Geometry check sheet. Reference: the model listing, model coordinates, mm. A direction names the side the tool comes from. Round coordinates to 2 decimals unless told otherwise and drop trailing zeros. Order: outer loops, then holes, each group sorted by start corner. A loop starts at its lowest first (then second) coordinate and runs counter-clockwise, first axis right, second up. Notation, with made-up numbers: (64.5, 13) -> (97.5, 13) arc R24 cw to (97.5, 44) -> close; hole circle Ø7 at (-4, 45.5). An arc over 180 degrees is marked (long way). Answer as a JSON object with one key per item and string values. Group by question number.
Autodesk Inventor part; units mm, degrees
ref_plane "YZ Plane" through (0, 0, 0) normal (1, 0, 0) x (0, 1, 0)
ref_plane "XZ Plane" through (0, 0, 0) normal (0, 1, 0) x (-1, 0, 0)
ref_plane "XY Plane" through (0, 0, 0) normal (0, 0, 1) x (1, 0, 0)
sketch "Sketch1" plane through (0, 0, 0) normal (0, 0, 1) x (1, 0, 0)
  line L0 (-35.56, 0) -> (35.56, 0) construction
  line L1 (0, -35.56) -> (0, 35.56) construction
  line L2 (-25.4, 25.4) -> (25.4, 25.4)
  line L3 (25.4, 25.4) -> (25.4, -25.4)
  line L4 (25.4, -25.4) -> (-25.4, -25.4)
  line L5 (-25.4, -25.4) -> (-25.4, 25.4)
  line L6 (-22.225, 22.225) -> (22.225, 22.225)
  line L7 (22.225, 22.225) -> (22.225, -22.225)
  line L8 (22.225, -22.225) -> (-22.225, -22.225)
  line L9 (-22.225, -22.225) -> (-22.225, 22.225)
  point P0 (0, 0)
  point P1 (-25.4, 0)
  point P2 (0, 25.4)
  point P3 (-22.225, 0)
  point P4 (0, 22.225)
  dimension "d0" = 50.8
  dimension "d1" = 3.175
  dimension "d11" = 50.8
  dimension "d12" = 3.175
extrude "Extrusion1" add sketch "Sketch1" along normal mid plane 101.6
sketch "Sketch6" plane through (-25.4, -25.4, 50.8) normal (-1, 0, 0) x (0, 0, 1)
  line L0 (-121.92, 25.4) -> (20.32, 25.4) construction
  line L1 (-50.8, -10.16) -> (-50.8, 60.96) construction
  line L2 (-71.8058, 50.8) -> (-29.7942, 50.8)
  line L3 (-29.7942, 50.8) -> (-29.7942, 0)
  line L4 (-29.7942, 0) -> (-71.8058, 0)
  line L5 (-71.8058, 0) -> (-71.8058, 50.8)
  line L6 (-101.6, 50.8) -> (0, 50.8) construction
  point P0 (-50.8, 25.4)
  point P1 (-71.8058, 25.4)
  point P2 (-50.8, 50.8)
  dimension "d23" = 42.0116
extrude "Extrusion7" cut sketch "Sketch6" against normal blind 3.175
sketch "Sketch7" plane through (-25.4, 25.4, 50.8) normal (0, 1, 0) x (1, 0, 0)
  circle A0 centre (37.35, 38.1) radius 2.0193 construction
  circle A1 centre (37.35, 63.5) radius 2.0193 construction
  circle A2 centre (37.35, 63.5) radius 2.413
  circle A3 centre (37.35, 38.1) radius 2.413
  point P0 (25.4, 50.8)
  dimension "d39" = 4.826
sketch "Sketch8" plane through (25.4, -25.4, 50.8) normal (1, 0, 0) x (0, 0, -1)
  line L0 (43.6, 4.4) -> (58, 4.4) construction
  line L1 (58, 4.4) -> (59.225, 3.175) construction
  line L2 (59.225, 3.175) -> (64.8, 3.175) construction
  line L3 (64.8, 9.4) -> (64.8, 3.175) construction
  arc A0 (66.8, 11.4) -> (64.8, 9.4) centre (66.8, 9.4) ccw construction
  line L4 (71.8, 11.4) -> (66.8, 11.4) construction
  line L5 (71.8, 11.4) -> (71.8, 45.4) construction
  arc A1 (71.8, 45.4) -> (70.8, 46.4) centre (50.8, 25.4) ccw construction
  line L6 (70.8, 46.4) -> (69, 46.4) construction
  line L7 (69, 46.4) -> (67.775, 47.625) construction
  line L8 (67.775, 47.625) -> (59.225, 47.625) construction
  line L9 (59.225, 47.625) -> (58, 46.4) construction
  line L10 (58, 46.4) -> (43.6, 46.4) construction
  line L11 (43.6, 46.4) -> (42.375, 47.625) construction
  line L12 (42.375, 47.625) -> (36.8, 47.625) construction
  line L13 (36.8, 41.4) -> (36.8, 47.625) construction
  arc A2 (34.8, 39.4) -> (36.8, 41.4) centre (34.8, 41.4) ccw construction
  line L14 (29.8, 39.4) -> (34.8, 39.4) construction
  line L15 (29.8, 39.4) -> (29.8, 5.4) construction
  arc A3 (29.8, 5.4) -> (30.8, 4.4) centre (50.8, 25.4) ccw construction
  line L16 (30.8, 4.4) -> (32.6, 4.4) construction
  line L17 (32.6, 4.4) -> (33.825, 3.175) construction
  line L18 (33.825, 3.175) -> (42.375, 3.175) construction
  line L19 (42.375, 3.175) -> (43.6, 4.4) construction
  circle A4 centre (50.8, 25.4) radius 14.195 construction
  circle A5 centre (32.8395, 7.4395) radius 2.0193 construction
  circle A6 centre (68.7605, 43.3605) radius 2.0193 construction
  circle A7 centre (50.8, 25.4) radius 6.985
  circle A8 centre (32.8395, 7.4395) radius 2.413
  circle A9 centre (68.7605, 43.3605) radius 2.413
  point P0 (50.8, 25.4)
  dimension "d28" = 13.97
  dimension "d36" = 4.826
sketch "Sketch9" plane through (-22.225, -22.225, 50.8) normal (1, 0, 0) x (0, 0, -1)
  circle A0 centre (86.7029, 6.35) radius 3.175 construction
  circle A1 centre (86.7029, 38.1) radius 3.175 construction
  circle A2 centre (14.8971, 6.35) radius 3.175 construction
  circle A3 centre (14.8971, 38.1) radius 3.175 construction
  circle A4 centre (86.7029, 6.35) radius 2.667
  circle A5 centre (14.8971, 6.35) radius 2.667
  circle A6 centre (86.7029, 38.1) radius 2.667
  circle A7 centre (14.8971, 38.1) radius 2.667
  point P0 (50.8, 22.225)
  dimension "d31" = 5.334
extrude "Extrusion10" cut sketch "Sketch9" against normal through all
sketch "Sketch10" plane through (25.4, -25.4, 50.8) normal (1, 0, 0) x (0, 0, -1)
  circle A0 centre (14.8971, 9.525) radius 3.175
  circle A1 centre (86.7029, 9.525) radius 3.175
  circle A2 centre (86.7029, 41.275) radius 3.175
  circle A3 centre (14.8971, 41.275) radius 3.175
  point P0 (50.8, 25.4)
extrude "Extrusion11" cut sketch "Sketch10" against normal up to next
extrude "Extrusion12" cut sketch "Sketch8" against normal up to next
extrude "Extrusion13" cut sketch "Sketch7" against normal through all
equation "\"d12\" = d1"
properties part number "Arm 4 inch" material "Aluminum 6061"
Item 1: Depth check by flat-ended pin: pin 1 Ø10 at (x, y) = (5.5, 14.5) entering from -Z. Enter the tip coordinate at first touch or a pass-through.
Item 2: Sectioned sample at B-B, the plane x = 1. Enter the section's corners in (y, z) (3 decimals), then the cut area to 3 significant figures.
Item 3: Thickness scan on L1, parallel to Y at x = -11, z = -13 (3 decimals); L2, parallel to Z at x = -23, y = -20. Record the ranges inside material, lowest first.
Item 4: Set-up check for faces 1 (the cylindrical face through (23.835, 16.015, 39.075)), 2 (the flat face through (0, -22.225, -1)), 3 (the flat face through (-22.225, 24, 0)): record each of +Z, -Z, +X, -X, +Y, -Y from which the full face is reachable in a straight line by a thin tool's end or side.
Item 5: Sectioned sample at C-C, the plane z = -23.5. Enter the section's corners in (x, y) (3 decimals), then the cut area to 3 significant figures.
Item 6: Mould release check, pull along X, two halves, no side actions. Record for faces 4 (the flat face through (-22.225, 0, 36)), 5 (the cylindrical face through (11.427, 23.835, -10.344)), 6 (the flat face through (-25.4, 0, 36)), 7 (the cylindrical face through (23.835, 6.926, 0.909)): pulls with the +X half, pulls with the -X half, needs draft (parallel to the pull), parting line crosses it, or undercut.
Item 7: Sectioned sample at A-A, the plane y = -9.5. Enter the section's corners in (x, z) (3 decimals).
Item 8: Sectioned sample at D-D, the plane y = 0. Enter the section's corners in (x, z) (3 decimals), then the cut area to 3 significant figures.
Result:
{
 "1": {"pin 1": "passes through"},
 "2": {"outline": "(-25.4, -50.8) -> (-22.225, -50.8) -> (-22.225, 50.8) -> (-25.4, 50.8) -> close; (22.225, -50.8) -> (25.4, -50.8) -> (25.4, 50.8) -> (22.225, 50.8) -> close", "area": "645 mm2"},
 "3": {"L1": "y = -25.4 to -22.225, 22.225 to 25.4", "L2": "z = -50.8 to -21.01, 21.01 to 50.8"},
 "4": {"face 1": "+X", "face 2": "+Z, -Z", "face 3": "-X, +Y, -Y"},
 "5": {"outline": "(-25.4, -25.4) -> (25.4, -25.4) -> (25.4, 25.4) -> (-25.4, 25.4) -> close; hole (-22.225, -22.225) -> (22.225, -22.225) -> (22.225, 22.225) -> (-22.225, 22.225) -> close", "area": "605 mm2"},
 "6": {"face 4": "undercut", "face 5": "undercut", "face 6": "pulls with the -X half", "face 7": "needs draft"},
 "7": {"outline": "(-25.4, -50.8) -> (-22.225, -50.8) -> (-22.225, -21.006) -> (-25.4, -21.006) -> close; (-25.4, 21.006) -> (-22.225, 21.006) -> (-22.225, 50.8) -> (-25.4, 50.8) -> close; (22.225, -50.8) -> (25.4, -50.8) -> (25.4, 50.8) -> (22.225, 50.8) -> close"},
 "8": {"outline": "(-25.4, -50.8) -> (-22.225, -50.8) -> (-22.225, -21.006) -> (-25.4, -21.006) -> close; (-25.4, 21.006) -> (-22.225, 21.006) -> (-22.225, 50.8) -> (-25.4, 50.8) -> close; (22.225, -50.8) -> (25.4, -50.8) -> (25.4, -6.985) -> (22.225, -6.985) -> close; (22.225, 6.985) -> (25.4, 6.985) -> (25.4, 50.8) -> (22.225, 50.8) -> close", "area": "467 mm2"}
}
